Autodesk Inventor part; units mm, degrees
ref_plane "YZ Plane" through (0, 0, 0) normal (1, 0, 0) x (0, 1, 0)
ref_plane "XZ Plane" through (0, 0, 0) normal (0, 1, 0) x (-1, 0, 0)
ref_plane "XY Plane" through (0, 0, 0) normal (0, 0, 1) x (1, 0, 0)
sketch "Sketch1" plane through (0, 0, 0) normal (0, 1, 0) x (-1, 0, 0)
  line L0 (-31.93, -49.55) -> (31.93, -49.55)
  line L1 (31.93, -49.55) -> (31.93, 49.55)
  line L2 (31.93, 49.55) -> (-31.93, 49.55)
  line L3 (-31.93, 49.55) -> (-31.93, -49.55)
  line L4 (-31.93, -49.55) -> (31.93, 49.55) construction
  line L5 (31.93, -49.55) -> (-31.93, 49.55) construction
  point P0 (0, 0)
  dimension "d0" = 63.86
  dimension "d1" = 99.1
extrude "Extrusion1" add sketch "Sketch1" along normal blind 5.08
sketch "Sketch2" plane through (0, 5.08, 0) normal (0, 1, 0) x (1, 0, 0)
  line L0 (28.73, 46.35) -> (-28.73, 46.35)
  line L1 (-28.73, 46.35) -> (-28.73, -46.35)
  line L2 (-28.73, -46.35) -> (28.73, -46.35)
  line L3 (28.73, -46.35) -> (28.73, 46.35)
  line L4 (28.73, 46.35) -> (-28.73, -46.35) construction
  line L5 (-28.73, 46.35) -> (28.73, -46.35) construction
  line L6 (-31.93, 49.55) -> (-31.93, -49.55)
  line L7 (-31.93, -49.55) -> (31.93, -49.55)
  line L8 (31.93, 49.55) -> (-31.93, 49.55)
  line L9 (31.93, -49.55) -> (31.93, 49.55)
  line L10 (25.53, -43.15) -> (31.93, -49.55) construction
  line L11 (23.0731, -46.35) -> (29.1016, -52.3784)
  line L12 (34.7584, -46.7216) -> (28.73, -40.6931)
  arc A0 (29.1016, -52.3784) -> (34.7584, -46.7216) centre (31.93, -49.55) ccw
  circle A1 centre (31.93, -49.55) radius 1.375
  point P0 (0, 0)
  dimension "d4" = 3.2
  dimension "d5" = 3.2
  dimension "d22" = 8
  dimension "d23" = 2.75
extrude "Extrusion2" add sketch "Sketch2" along normal blind 48 contours L0 L1 L2 L11 L7 L6 L8 L9 L12 L3 | L12 L9 A1 L7 L11 L2 L3 | L9 L7 A1 picked at (31.2859, -48.9059)
sketch "Sketch3" plane through (0, 5.08, 0) normal (0, 1, 0) x (1, 0, 0)
  line L0 (28.73, -46.35) -> (-28.73, -46.35) construction
  line L1 (0, -46.35) -> (0, 46.35) construction
  line L2 (28.73, 46.35) -> (-28.73, 46.35) construction
  circle A0 centre (-24.5, -36.35) radius 3.5
  circle A1 centre (-24.5, -36.35) radius 1.375
  line L3 (28.73, 46.35) -> (28.73, -46.35) construction
  line L4 (28.73, 0) -> (-28.73, 0) construction
  line L5 (-28.73, -46.35) -> (-28.73, 46.35) construction
  circle A2 centre (-24.5, 21.65) radius 3.5
  circle A3 centre (-24.5, 21.65) radius 1.375
  circle A4 centre (24.5, -36.35) radius 3.5
  circle A5 centre (24.5, -36.35) radius 1.375
  circle A6 centre (24.5, 21.65) radius 3.5
  circle A7 centre (24.5, 21.65) radius 1.375
  point P0 (0, 0)
  dimension "d8" = 7
  dimension "d9" = 2.75
  dimension "d10" = 10
  dimension "d11" = 24.5
  dimension "d14" = 58
extrude "Extrusion3" add sketch "Sketch3" along normal blind 5
sketch "Sketch4" plane through (0, 0, 0) normal (0, -1, 0) x (1, 0, 0)
  line L0 (29.6707, 47.5763) -> (34.1893, 51.5237) construction
  line L1 (31.93, 49.55) -> (31.93, -49.55)
  line L2 (31.93, 43.5747) -> (37.1499, 48.1348)
  line L3 (31.2287, 54.9127) -> (26.7101, 50.9652)
  arc A0 (26.7101, 50.9652) -> (25.6267, 49.55) centre (29.6707, 47.5763) ccw
  arc A1 (37.1499, 48.1348) -> (31.2287, 54.9127) centre (34.1893, 51.5237) ccw
  line L4 (-31.93, 49.55) -> (31.93, 49.55)
  line L5 (25.6267, 49.55) -> (31.93, 49.55)
  line L6 (31.93, 49.55) -> (31.93, 43.5747)
  circle A2 centre (34.1893, 51.5237) radius 1.85
  line L7 (0, 49.55) -> (0, -49.55) construction
  line L8 (31.93, -49.55) -> (-31.93, -49.55) construction
  line L9 (31.93, 0) -> (-33.3, 0) construction
  line L10 (31.93, -49.55) -> (31.93, 49.55)
  line L11 (31.93, -43.5747) -> (37.1499, -48.1348)
  line L12 (31.2287, -54.9127) -> (26.7101, -50.9652)
  arc A3 (25.6267, -49.55) -> (26.7101, -50.9652) centre (29.6707, -47.5763) ccw
  arc A4 (31.2287, -54.9127) -> (37.1499, -48.1348) centre (34.1893, -51.5237) ccw
  line L13 (-31.93, -49.55) -> (31.93, -49.55)
  circle A5 centre (34.1893, -51.5237) radius 1.85
  line L14 (-31.93, 49.55) -> (-31.93, -49.55)
  line L15 (-31.93, 43.5747) -> (-37.1499, 48.1348)
  line L16 (-31.2287, 54.9127) -> (-26.7101, 50.9652)
  arc A6 (-25.6267, 49.55) -> (-26.7101, 50.9652) centre (-29.6707, 47.5763) ccw
  arc A7 (-31.2287, 54.9127) -> (-37.1499, 48.1348) centre (-34.1893, 51.5237) ccw
  line L17 (-25.6267, 49.55) -> (-31.93, 49.55)
  circle A8 centre (-34.1893, 51.5237) radius 1.85
  arc A9 (-37.1499, -48.1348) -> (-31.2287, -54.9127) centre (-34.1893, -51.5237) ccw
  line L18 (-31.93, -43.5747) -> (-37.1499, -48.1348)
  line L19 (-31.2287, -54.9127) -> (-26.7101, -50.9652)
  arc A10 (-26.7101, -50.9652) -> (-25.6267, -49.55) centre (-29.6707, -47.5763) ccw
  circle A11 centre (-34.1893, -51.5237) radius 1.85
  line L20 (-25.6267, -49.55) -> (-31.93, -49.55)
  line L21 (-31.93, -49.55) -> (-31.93, 49.55)
  point P0 (0, 0)
  point P1 (-31.93, -43.5747)
  point P2 (31.93, -43.5747)
  point P3 (31.93, -49.55)
  dimension "d24" = 3
  dimension "d25" = 9
  dimension "d26" = 131.141
  dimension "d27" = 3.7
extrude "Extrusion4" add sketch "Sketch4" against normal up to surface (53.08 mm away) contours L4 A0 L3 A1 L2 L1 | L11 A4 L12 A3 L13 L1 | L4 L14 L15 A7 L16 A6 | A10 L19 A9 L18 L14 L13
fillet "Fillet2" radius 2 4 edges at (28.73, 29.08, -46.35) (-28.73, 29.08, -46.35) (-28.73, 29.08, 46.35) (28.73, 29.08, 46.35)
sketch "Sketch5" plane through (0, 5.08, 0) normal (0, 1, 0) x (1, 0, 0)
  line L0 (15, 0) -> (-15, 0) construction
  line L1 (15, 2.5) -> (-15, 2.5)
  line L2 (-15, -2.5) -> (15, -2.5)
  arc A0 (15, -2.5) -> (15, 2.5) centre (15, 0) ccw
  arc A1 (-15, 2.5) -> (-15, -2.5) centre (-15, 0) ccw
  line L3 (-26.73, -46.35) -> (26.73, -46.35) construction
  line L4 (0, -46.35) -> (0, 46.35) construction
  line L5 (-26.73, 46.35) -> (26.73, 46.35) construction
  arc A2 (-15, 12.5) -> (-15, 7.5) centre (-15, 10) ccw
  line L6 (15, 12.5) -> (-15, 12.5)
  line L7 (-15, 7.5) -> (15, 7.5)
  arc A3 (15, 7.5) -> (15, 12.5) centre (15, 10) ccw
  arc A4 (-15, 22.5) -> (-15, 17.5) centre (-15, 20) ccw
  line L8 (15, 22.5) -> (-15, 22.5)
  line L9 (-15, 17.5) -> (15, 17.5)
  arc A5 (15, 17.5) -> (15, 22.5) centre (15, 20) ccw
  arc A6 (-15, 32.5) -> (-15, 27.5) centre (-15, 30) ccw
  line L10 (15, 32.5) -> (-15, 32.5)
  line L11 (-15, 27.5) -> (15, 27.5)
  arc A7 (15, 27.5) -> (15, 32.5) centre (15, 30) ccw
  arc A8 (-15, -7.5) -> (-15, -12.5) centre (-15, -10) ccw
  line L12 (-15, -12.5) -> (15, -12.5)
  line L13 (15, -7.5) -> (-15, -7.5)
  arc A9 (15, -12.5) -> (15, -7.5) centre (15, -10) ccw
  arc A10 (-15, -17.5) -> (-15, -22.5) centre (-15, -20) ccw
  line L14 (-15, -22.5) -> (15, -22.5)
  line L15 (15, -17.5) -> (-15, -17.5)
  arc A11 (15, -22.5) -> (15, -17.5) centre (15, -20) ccw
  arc A12 (-15, -27.5) -> (-15, -32.5) centre (-15, -30) ccw
  line L16 (-15, -32.5) -> (15, -32.5)
  line L17 (15, -27.5) -> (-15, -27.5)
  arc A13 (15, -32.5) -> (15, -27.5) centre (15, -30) ccw
  point P0 (0, 0)
  dimension "d31" = 15
  dimension "d32" = 5
  dimension "d35" = 10
  dimension "d42" = 10
extrude "Extrusion5" cut sketch "Sketch5" against normal up to surface (5.08 mm away)
sketch "Sketch12" plane through (31.93, 0, 43.5747) normal (1, 0, 0) x (0, 0, -1)
  line L0 (0, 53.08) -> (0, 0)
  line L1 (28.1666, 16.69) -> (28.1666, 14.2116)
  line L2 (43.1666, 14.2116) -> (43.1666, 16.69)
  line L3 (10.2763, 12.8971) -> (10.2763, 13.09)
  line L4 (18.257, 13.09) -> (18.257, 12.8971)
  line L5 (53.7666, 17.41) -> (53.7666, 11.41)
  line L6 (60.7666, 11.41) -> (60.7666, 17.41)
  line L7 (11.2666, 14.1354) -> (17.2666, 14.1354)
  line L8 (21.0747, 5.08) -> (26.0747, 5.08)
  line L9 (26.0747, 5.08) -> (21.0747, 5.08)
  line L10 (41.0747, 5.08) -> (46.0747, 5.08)
  line L11 (46.0747, 5.08) -> (41.0747, 5.08)
  line L12 (51.0747, 5.08) -> (56.0747, 5.08)
  line L13 (56.0747, 5.08) -> (51.0747, 5.08)
  line L14 (61.0747, 5.08) -> (66.0747, 5.08)
  line L15 (66.0747, 5.08) -> (61.0747, 5.08)
  line L16 (11.0747, 5.08) -> (16.0747, 5.08)
  line L17 (16.0747, 5.08) -> (11.0747, 5.08)
  line L18 (31.0747, 5.08) -> (36.0747, 5.08)
  line L19 (36.0747, 5.08) -> (31.0747, 5.08)
  line L20 (71.0747, 5.08) -> (76.0747, 5.08)
  line L21 (76.0747, 5.08) -> (71.0747, 5.08)
  line L22 (3.7247, 5.08) -> (10.7247, 5.08)
  line L23 (3.7247, 5.08) -> (10.7247, 5.08)
  line L24 (61.7247, 5.08) -> (68.7247, 5.08)
  line L25 (61.7247, 5.08) -> (68.7247, 5.08)
  line L26 (-2.7753, 5.08) -> (-0.7753, 5.08)
  line L27 (-0.7753, 5.08) -> (87.9247, 5.08)
  line L28 (87.9247, 5.08) -> (89.9247, 5.08)
  line L29 (89.9247, 5.08) -> (87.9247, 5.08)
  line L30 (87.9247, 5.08) -> (-0.7753, 5.08)
  line L31 (-0.7753, 5.08) -> (-2.7753, 5.08)
  line L32 (5.8497, 10.08) -> (8.5997, 10.08)
  line L33 (10.2763, 12.9936) -> (18.257, 12.9936) construction
  line L34 (14.2666, 14.1354) -> (14.2666, 12.9936) construction
  line L35 (7.2763, 19.08) -> (21.257, 19.08)
  line L36 (21.257, 19.08) -> (21.257, 10.08)
  line L37 (21.257, 10.08) -> (7.2763, 10.08)
  line L38 (7.2763, 10.08) -> (7.2763, 19.08)
  line L39 (42.3666, 17.49) -> (28.9666, 17.49)
  line L40 (47.1666, 10.08) -> (24.1666, 10.08)
  line L41 (24.1666, 10.08) -> (24.1666, 22.08)
  line L42 (24.1666, 22.08) -> (47.1666, 22.08)
  line L43 (47.1666, 22.08) -> (47.1666, 10.08)
  line L44 (60.7666, 17.41) -> (57.2666, 17.41)
  line L45 (63.7666, 10.08) -> (50.7666, 10.08)
  line L46 (50.7666, 10.08) -> (50.7666, 19.68)
  line L47 (50.7666, 19.68) -> (63.7666, 19.68)
  line L48 (63.7666, 19.68) -> (63.7666, 10.08)
  point P0 (43.5747, 0)
  dimension "d99" = 3
  dimension "d100" = 3
  dimension "d101" = 0
  dimension "d102" = 9
  dimension "d103" = 4
  dimension "d104" = 4
  dimension "d105" = 0
  dimension "d106" = 12
  dimension "d108" = 3
  dimension "d109" = 3
  dimension "d110" = 0
  dimension "d111" = 9.6
extrude "Extrusion9" cut sketch "Sketch12" against normal up to surface (3.2 mm away)
sketch "Sketch14" plane through (25.6267, 0, -49.55) normal (0, 0, -1) x (-1, 0, 0)
  line L0 (0.5198, 11.61) -> (0.5198, 25.11)
  line L1 (16.3998, 11.61) -> (16.3998, 25.11)
  line L2 (0.5198, 25.11) -> (16.3998, 25.11)
  line L3 (0.5198, 11.61) -> (16.3998, 11.61)
  line L4 (0.5198, 18.36) -> (16.3998, 18.36) construction
  line L5 (16.8998, 11.11) -> (0.2698, 11.11)
  line L6 (0.2698, 11.11) -> (0.2698, 25.61)
  line L7 (0.2698, 25.61) -> (16.8998, 25.61)
  line L8 (16.8998, 25.61) -> (16.8998, 11.11)
  line L9 (24.2098, 27.1) -> (30.2098, 27.1)
  line L10 (34.7598, 21.3896) -> (34.7598, 18.3896)
  line L11 (19.6598, 18.3896) -> (19.6598, 21.3896)
  line L12 (25.6198, 11.41) -> (28.7998, 11.41)
  line L13 (35.2598, 10.91) -> (18.6659, 10.91)
  line L14 (18.6659, 10.91) -> (18.6659, 28.1)
  line L15 (18.6659, 28.1) -> (35.2598, 28.1)
  line L16 (35.2598, 28.1) -> (35.2598, 10.91)
  line L17 (19.1659, 18.3896) -> (19.1659, 21.3896)
  point P0 (25.6267, 0)
  dimension "d114" = 0.5
  dimension "d115" = 0.5
  dimension "d116" = 0.25
  dimension "d117" = 0.5
  dimension "d120" = 1
  dimension "d122" = 0.5
  dimension "d123" = 0.5
  dimension "d124" = 0.5
extrude "Extrusion10" cut sketch "Sketch14" against normal up to surface (3.2 mm away) contours L0 L2 L1 L3 | L13 L14 L15 L16
properties part number "Test" material "ABS Plastic"
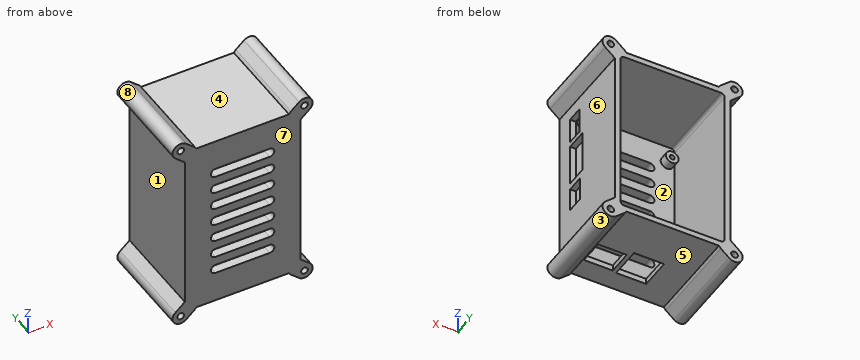
Verification items for the finished model (mm, model axes). Face numbers are marked on the shaded views. A direction names the side the tool comes from. Round coordinates to 2 decimals unless told otherwise and drop trailing zeros. Loops run counter-clockwise (first coordinate to the right, second up) from the corner with the lowest first, then second, coordinate; pieces in that order, holes last. Notation, with made-up numbers: (87, -11.75) - (115, -11.75) arc R24 cw to (115, 26.25) - close; hole circle Ø4 at (-25, 8.25). An arc over 180 degrees is marked (long way). Use a Markdown table: item, result. Add a question column.
1. Section check C-C, the plane y = 50.5. Give the number of separate pieces and of enclosed holes in the cut face, plus the area to 3 significant figures.
2. Thickness scan on probe 1 along Z at (x, y) = (-24.5, 7.9) (3 decimals); probe 2 along X at (y, z) = (8.05, -21.65) (3 decimals); probe 3 along Z at (x, y) = (-15, 50). Record the ranges inside material, lowest first. Write a range as [from, to].
3. Gauge pin test, flat ends, axial feed: pin 1 (10 mm diameter, centred on x = 8.5, z = 2.5, fed in from +Y); pin 2 (24 mm diameter, centred on x = 0, y = 34, fed in from -Z); pin 3 (1.6 mm diameter, centred on y = 23, z = -48, fed in from +X); pin 4 (3.5 mm diameter, centred on x = -34.19, z = 51.52, fed in from +Y). Record the tip position at first contact, or that the pin passes through.
4. Access from +Z, -Z, +X, -X, +Y, -Y to the whole of each face (thin tool, end or side, straight path). Record for the marked faces 1, 2, 3, 4 and 5.
5. Section check A-A, the plane z = -30. Record the boundary of the cut face in (x, y), plus the area to 3 significant figures.
6. Release check for a two-part mould opening along X. For the marked faces 6, 7 and 8 record: released by +X, released by -X, zero draft, split by the parting line, or undercut.
7. Section check B-B, the plane z = -10. Record the boundary of the cut face in (x, y), plus the area to 3 significant figures.
Checks:
| question | item | result |
|---|---|---|
| 1 | separate pieces | 1 |
| 1 | enclosed holes | 5 |
| 1 | area | 1,280 mm^2 |
| 2 | probe 1 | z = [-49.55, -46.35], [-25.15, -23.025], [-20.275, -18.15], [32.85, 34.975], [37.725, 39.85], [46.35, 49.55] |
| 2 | probe 2 | x = [-31.93, -28.73], [-28, -25.875], [-23.125, -21], [21, 23.125], [25.875, 28], [28.73, 31.93] |
| 2 | probe 3 | z = [-49.55, -46.35], [46.35, 49.55] |
| 3 | pin 1 | stops at y = 5.08 |
| 3 | pin 2 | stops at z = -49.55 |
| 3 | pin 3 | stops at x = 37.77 |
| 3 | pin 4 | passes through |
| 4 | face 1 | -X, +Y, -Y |
| 4 | face 2 | +Y |
| 4 | face 3 | +Y, -Y |
| 4 | face 4 | +Z, +Y, -Y |
| 4 | face 5 | -Z, +Y, -Y |
| 5 | outline | (-31.93, 0) - (-17.5, 0) - (-17.5, 5.08) - (-28.73, 5.08) - (-28.73, 53.08) - (-31.93, 53.08) - close; (17.5, 0) - (31.93, 0) - (31.93, 53.08) - (28.73, 53.08) - (28.73, 5.08) - (17.5, 5.08) - close |
| 5 | area | 454 mm^2 |
| 6 | face 6 | released by +X |
| 6 | face 7 | zero draft |
| 6 | face 8 | undercut |
| 7 | outline | (-31.93, 0) - (-17.5, 0) - (-17.5, 5.08) - (-28.73, 5.08) - (-28.73, 53.08) - (-31.93, 53.08) - close; (17.5, 0) - (31.93, 0) - (31.93, 10.08) - (28.73, 10.08) - (28.73, 5.08) - (17.5, 5.08) - close; (28.73, 19.68) - (31.93, 19.68) - (31.93, 53.08) - (28.73, 53.08) - close |
| 7 | area | 423 mm^2 |
